CAD build for the part. Positions are in the model's coordinates, mm. A direction names the side the tool comes from. Round coordinates to 2 decimals unless told otherwise and drop trailing zeros. Loops run counter-clockwise (first coordinate to the right, second up) from the corner with the lowest first, then second, coordinate; pieces in that order, holes last. Notation, with made-up numbers: (32.25, 83) -> (48.25, 83) arc R30 cw to (48.25, 114) -> close; hole circle Ø5 at (80, -31). An arc over 180 degrees is marked (long way). Answer as CSV lines item,"result".
```python
from build123d import *

# Parameters (mm, degrees)
SKETCH_W        = 100
SKETCH_H        = 100
PAD_DEPTH       = 15
FILLET_R        = 20
POCKET_DEPTH    = 3
POCKET001_DEPTH = 10
SKETCH003_R     = 2.2
POCKET002_DEPTH = 12.001
SKETCH004_R     = 5
POCKET003_DEPTH = 2.001


with BuildPart() as part:
    # Sketch → Pad (new body)
    with BuildSketch(Plane.XY):
        Rectangle(SKETCH_W, SKETCH_H)
    extrude(amount=PAD_DEPTH)

    # Fillet
    fillet_edges = [part.edges().sort_by_distance(p)[0] for p in [
        (-50, 50, 7.5),
        (50, 50, 7.5),
        (50, -50, 7.5),
        (-50, -50, 7.5),
    ]]
    fillet(fillet_edges, radius=FILLET_R)

    # Sketch001 (on Face5 of Fillet) → Pocket (cut)
    with BuildSketch(Plane.XY.offset(15)):
        with BuildLine():
            Line((-30, 47), (30, 47))
            ThreePointArc((47, 30), (42.020815, 42.020815), (30, 47))
            Line((47, 30), (47, -30))
            ThreePointArc((30, -47), (42.020815, -42.020815), (47, -30))
            Line((30, -47), (-30, -47))
            ThreePointArc((-47, -30), (-42.020815, -42.020815), (-30, -47))
            Line((-47, -30), (-47, 30))
            ThreePointArc((-30, 47), (-42.020815, 42.020815), (-47, 30))
        make_face()
    extrude(amount=-POCKET_DEPTH, mode=Mode.SUBTRACT)

    # Sketch002 (on Face19 of Pocket) → Pocket001 (cut)
    with BuildSketch(Plane.XY.offset(12)):
        with BuildLine():
            Line((35, 44.99997), (35, 34.99997))
            Line((35, 34.99997), (45, 34.99997))
            Line((45, 34.99997), (45, -29.99997))
            ThreePointArc((30, -44.99997), (40.606602, -40.606572), (45, -29.99997))
            Line((30, -44.99997), (-35, -44.99997))
            Line((-35, -44.99997), (-35, -34.99997))
            Line((-35, -34.99997), (-45, -34.99997))
            Line((-45, -34.99997), (-45, 29.99997))
            ThreePointArc((-30, 44.99997), (-40.606602, 40.606572), (-45, 29.99997))
            Line((-30, 44.99997), (35, 44.99997))
        make_face()
    extrude(amount=-POCKET001_DEPTH, mode=Mode.SUBTRACT)

    # Sketch003 (on Face19 of Pocket001) → Pocket002 (cut, through all)
    with BuildSketch(Plane.XY.offset(12)):
        with Locations((-40, -40)):
            Circle(SKETCH003_R)
        with Locations((40, 40)):
            Circle(SKETCH003_R)
    extrude(amount=-POCKET002_DEPTH, mode=Mode.SUBTRACT)

    # Sketch004 (on Face32 of Pocket002) → Pocket003 (cut, through all)
    with BuildSketch(Plane.XY.offset(2)):
        Circle(SKETCH004_R)
    extrude(amount=-POCKET003_DEPTH, mode=Mode.SUBTRACT)


solid = part.part
```
Q1. Two-plate mould, pull along Y, no slides. Class faces 3 (the cylindrical face through (43.986, -44.297, 7.605)), 4 (the cylindrical face through (-1.08, -4.88, 1.01)), 5 (the cylindrical face through (-41.89, 42.15, 13.52)), 6 (the flat face through (0, 50, 7)): pulls with the +Y half, pulls with the -Y half, needs draft (parallel to the pull), parting line crosses it, or undercut.
Results:
face 3,"pulls with the -Y half"
face 4,"undercut"
face 5,"undercut"
face 6,"pulls with the +Y half"
Q2. Slice it at A-A, the plane y = 0. Give the cut face in (x, z), and give its area (3 significant figures).
Results:
outline,"(-50, 0) -> (-5, 0) -> (-5, 2) -> (-45, 2) -> (-45, 12) -> (-47, 12) -> (-47, 15) -> (-50, 15) -> close; (5, 0) -> (50, 0) -> (50, 15) -> (47, 15) -> (47, 12) -> (45, 12) -> (45, 2) -> (5, 2) -> close"
area,"298 mm2"
Q3. Slice it at C-C, the plane z = 9.25. Give the cut face in (x, y).
Results:
outline,"(-50, -30) arc R20 ccw to (-30, -50) -> (30, -50) arc R20 ccw to (50, -30) -> (50, 30) arc R20 ccw to (30, 50) -> (-30, 50) arc R20 ccw to (-50, 30) -> close; hole (-45, -35) -> (-35, -35) -> (-35, -45) -> (30, -45) arc R15 ccw to (45, -30) -> (45, 35) -> (35, 35) -> (35, 45) -> (-30, 45) arc R15 ccw to (-45, 30) -> close; hole circle Ø4.4 at (-40, -40); hole circle Ø4.4 at (40, 40)"
Q4. Probe L1, parallel to Y at x = 20, z = 13; L2, parallel to Y at x = 27.5, z = 7.25. List the from-to ranges inside material, lowest first. Write a range as [from, to].
Results:
L1,"[-50, -47], [47, 50]"
L2,"[-50, -45], [45, 50]"
Q5. Drop flat-ended pins along their axis: pin 1 Ø6 at (x, y) = (0, 0) entering from +Z; pin 2 Ø8 at (x, z) = (-37.5, 6.5) entering from +Y; pin 3 Ø8 at (x, z) = (38, 7) entering from -Y; pin 4 Ø1.5 at (x, y) = (-28, -39.5) entering from +Z. Give the stop position or say it passes through.
Results:
pin 1,"through"
pin 2,"y = 49.69"
pin 3,"y = -49.6"
pin 4,"z = 2"
Q6. Slice it at D-D, the plane x = 24.5. Give the cut face in (y, z), and give its area (3 significant figures).
Results:
outline,"(-50, 0) -> (50, 0) -> (50, 15) -> (47, 15) -> (47, 12) -> (45, 12) -> (45, 2) -> (-45, 2) -> (-45, 12) -> (-47, 12) -> (-47, 15) -> (-50, 15) -> close"
area,"318 mm2"
Q7. Tool access for faces 1 (the cylindrical face through (-44.297, 43.986, 7.605)), 2 (the flat face through (-47, 0, 14)): list every direction of +Z, -Z, +X, -X, +Y, -Y with a clear straight run to the whole face (end or side of a thin tool).
Results:
face 1,"+Z, -Z, -X, +Y"
face 2,"+Z"
